from build123d import *

# Parameters (mm, degrees)
SKETCH1_W           = 20
SKETCH1_H           = 20
BOSS_EXTRUDE1_DEPTH = 16
FILLET1_R           = 1
CHAMFER1_SIZE       = 0.4


with BuildPart() as part:
    # Sketch1 → Boss-Extrude1 (new body)
    with BuildSketch(Plane.XY):
        Rectangle(SKETCH1_W, SKETCH1_H)
    extrude(amount=BOSS_EXTRUDE1_DEPTH)

    # Sketch4 → CBORE for M5 Hex Socket Head Cap Screw1 (revolve, cut)
    with BuildSketch(Plane(origin=(0, 10, 8), x_dir=(0, 0, 1), z_dir=(1, 0, 0))):
        Polygon((0, 0), (0, 20), (2.75, 20), (2.75, 11), (5, 11), (5, 0.025), (5.025, 0), align=None)
    revolve(axis=Axis((0, 16.35, 8), (0, -1, 0)), mode=Mode.SUBTRACT)

    # Fillet1
    fillet1_edges = [part.edges().sort_by_distance(p)[0] for p in [
        (10, 0, 16),
        (-10, 0, 16),
        (10, 0, 0),
        (-10, 0, 0),
    ]]
    fillet(fillet1_edges, radius=FILLET1_R)

    # Chamfer1
    chamfer1_edges = [part.edges().sort_by_distance(p)[0] for p in [
        (10, 10, 8),
        (10, -10, 8),
        (0, 10, 0),
        (-10, 10, 8),
        (0, 10, 16),
        (-9.707106781, 10, 15.707106781),
        (-9.707106781, 10, 0.292893219),
        (9.707106781, 10, 15.707106781),
        (9.707106781, 10, 0.292893219),
        (0, -10, 0),
        (0, -10, 16),
        (-10, -10, 8),
        (-9.707106781, -10, 15.707106781),
        (-9.707106781, -10, 0.292893219),
        (9.707106781, -10, 15.707106781),
        (9.707106781, -10, 0.292893219),
    ]]
    chamfer(chamfer1_edges, length=CHAMFER1_SIZE)


solid = part.part
Source: CAD feature listing. Evaluate the final solid. Frame: model axes, mm. Round coordinates to 2 decimals unless told otherwise and drop trailing zeros. Loops run counter-clockwise (first coordinate to the right, second up) from the corner with the lowest first, then second, coordinate; pieces in that order, holes last. Notation, with made-up numbers: (59, 86) -> (77, 86) arc R27 ccw to (77, 119) -> close; hole circle Ø1 at (77, 35.25). An arc over 180 degrees is marked (long way). Answer as a JSON object with one key per item and string values. Group by question number.
Q1. Section query B-B (y = 8.75). Output: boundary loops of the cut face in (x, z), plus the area to 3 significant figures.
Q2. Section query A-A (z = 8). Output: boundary loops of the cut face in (x, y) (3 decimals).
Q3. Ray query, line 1 (Z direction, x = 0, y = -8); line 2 (X direction, y = -3, z = 8); line 3 (X direction, y = 4.75, z = 8). Return the intervals inside material, ascending. Write a range as from..to.
Q4. Contact query for a flat-ended pin moving along its axis: P1, Ø5, axis at x = -2, z = 7.5, coming from the +Y side. Output: stop coordinate, or through.
Q5. Mould query, pull axis Z, two halves, no side actions, for faces 1 (the conical face through (9.53, 9.842, 0.458)), 2 (the flat face through (2.2, -1, 5.8)), 3 (the flat face through (0, 0, 16)). Classes: pulls with the +Z half, pulls with the -Z half, needs draft (parallel to the pull), parting line crosses it, or undercut.
Q6. Section query D-D (y = -8.5). Output: boundary loops of the cut face in (x, z).
Q7. Section query C-C (x = 0). Output: boundary loops of the cut face in (y, z) (3 decimals), plus the area to 3 significant figures.
Completed:
{
 "1": {"outline": "(-10, 1) arc R1 ccw to (-9, 0) -> (9, 0) arc R1 ccw to (10, 1) -> (10, 15) arc R1 ccw to (9, 16) -> (-9, 16) arc R1 ccw to (-10, 15) -> close; hole circle Ø10 at (0, 8)", "area": "241 mm²"},
 "2": {"outline": "(-10, -9.6) -> (-9.6, -10) -> (-2.75, -10) -> (-2.75, -1) -> (-5, -1) -> (-5, 9.975) -> (-5.025, 10) -> (-9.6, 10) -> (-10, 9.6) -> close; (2.75, -10) -> (9.6, -10) -> (10, -9.6) -> (10, 9.6) -> (9.6, 10) -> (5.025, 10) -> (5, 9.975) -> (5, -1) -> (2.75, -1) -> close"},
 "3": {"line 1": "0..5.25, 10.75..16", "line 2": "-10..-2.75, 2.75..10", "line 3": "-10..-5, 5..10"},
 "4": {"P1": "y = -1"},
 "5": {"face 1": "pulls with the -Z half", "face 2": "undercut", "face 3": "pulls with the +Z half"},
 "6": {"outline": "(-10, 1) arc R1 ccw to (-9, 0) -> (9, 0) arc R1 ccw to (10, 1) -> (10, 15) arc R1 ccw to (9, 16) -> (-9, 16) arc R1 ccw to (-10, 15) -> close; hole circle Ø5.5 at (0, 8)"},
 "7": {"outline": "(-10, 0.4) -> (-9.6, 0) -> (9.6, 0) -> (10, 0.4) -> (10, 2.975) -> (9.975, 3) -> (-1, 3) -> (-1, 5.25) -> (-10, 5.25) -> close; (-10, 10.75) -> (-1, 10.75) -> (-1, 13) -> (9.975, 13) -> (10, 13.025) -> (10, 15.6) -> (9.6, 16) -> (-9.6, 16) -> (-10, 15.6) -> close", "area": "160 mm²"}
}
